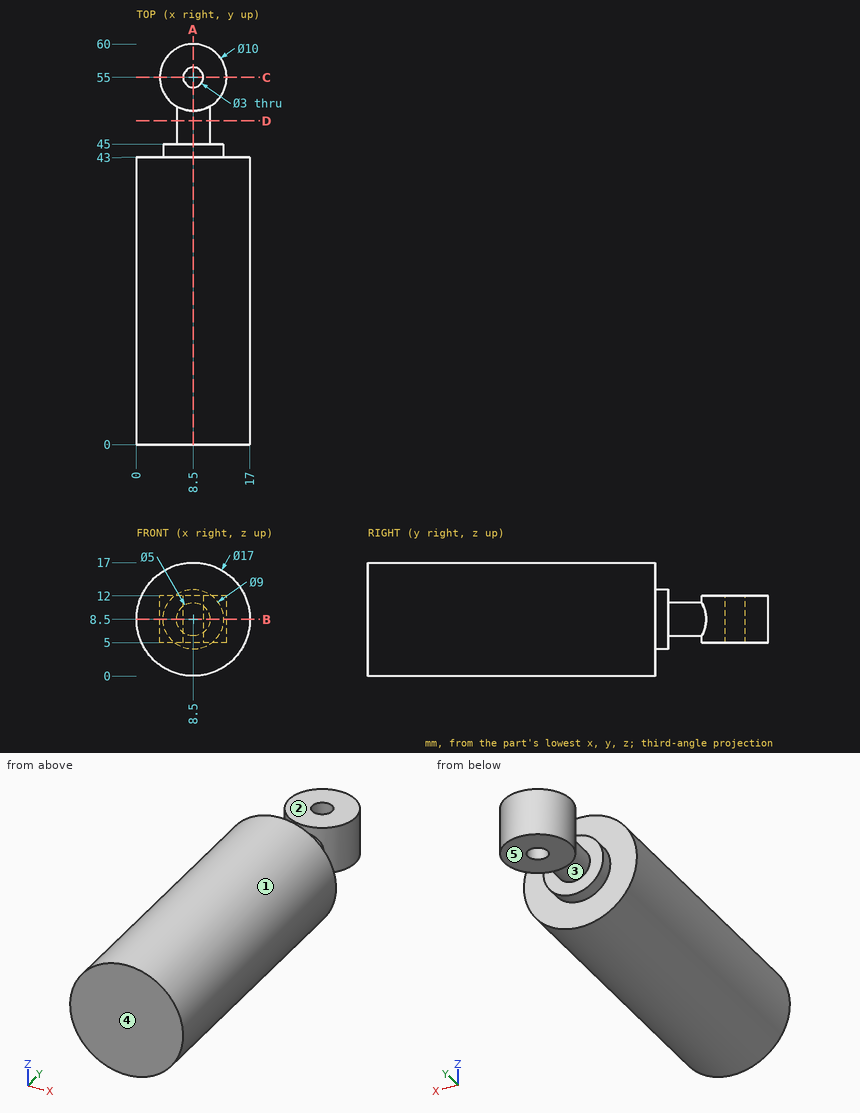
Study the drawing (mm; zero at the part's minimum x, y, z) and answer. A direction names the side the tool comes from. Give positions to 0.01 mm unless a question says otherwise; leave off trailing zeros. Write each loop counter-clockwise with the first axis right and the second up, starting at its lowest first coordinate (ties: lowest second). Pieces come first, ordered by that corner, then holes. Notation, with made-up numbers: (-36.5, 37) - (2.5, 37) arc R12 ccw to (2.5, 45) - close; hole circle Ø2 at (17.25, 69). An arc over 180 degrees is marked (long way). Write item = value, one per line. Start each with the question number.
Item 1: A tool of negligible diameter and unlimited length cuts with its end or side. For the marked faces 1 and 2, from which of +Z, -Z, +X, -X, +Y, -Y can it reach the whole face along a straight path? Write none if from no direction.
Item 2: Find section A-A (x = 8.5). Give the vertices of the cut face in (y, z), then the cut area to 3 significant figures.
Item 3: Each of these flat-tipped pins is pushed along its axis until it touches: P1, Ø3, axis at x = 10, y = 54.5, coming from the -Z side; P2, Ø5, axis at x = 8.5, y = 54, coming from the +Z side; P3, Ø2, axis at y = 27, z = 14.5, coming from the -X side. Where does it stop, or does it pass through?
Item 4: The mould has two halves that part along Y. Classify the marked faces 3, 4 and 5: +Y half, -Y half, draft (parallel to the pull), parting line (faces both ways), or undercut.
Item 5: Find section B-B (z = 8.5). Give the vertices of the cut face in (x, y), then the cut area to 3 significant figures.
Item 6: Find the intervals of material crossed by probe 1 along Y at (x, z) = (8.5, 9.5); probe 2 along Y at (x, z) = (5.5, 11.25); probe 3 along Y at (x, z) = (12, 13.25), in increasing order. Write a range as [from, to].
Item 7: Find section C-C (y = 55). Give the vertices of the cut face in (x, z), then the cut area to 3 significant figures.
Item 8: Find section D-D (y = 48.5). Give the vertices of the cut face in (x, z), then the cut area to 3 significant figures.
Response:
q1.face_1 = +Y, -Y
q1.face_2 = +Z, +X, -X, +Y
q2.outline = (0, 0) - (43, 0) - (43, 4) - (45, 4) - (45, 6) - (50, 6) - (50, 5) - (53.5, 5) - (53.5, 12) - (50, 12) - (50, 11) - (45, 11) - (45, 13) - (43, 13) - (43, 17) - (0, 17) - close; (56.5, 5) - (60, 5) - (60, 12) - (56.5, 12) - close
q2.area = 823 mm²
q3.P1 = 5
q3.P2 = 12
q3.P3 = 1.63
q4.face_3 = undercut
q4.face_4 = -Y half
q4.face_5 = draft
q5.outline = (0, 0) - (17, 0) - (17, 43) - (13, 43) - (13, 45) - (11, 45) - (11, 50.67) arc R5 ccw (long way) to (6, 50.67) - (6, 45) - (4, 45) - (4, 43) - (0, 43) - close; hole circle Ø3 at (8.5, 55)
q5.area = 847 mm²
q6.probe_1 = [0, 53.5], [56.5, 60]
q6.probe_2 = [0, 45], [51, 59]
q6.probe_3 = [0, 43]
q7.outline = (3.5, 5) - (7, 5) - (7, 12) - (3.5, 12) - close; (10, 5) - (13.5, 5) - (13.5, 12) - (10, 12) - close
q7.area = 49.0 mm²
q8.outline = circle Ø5 at (8.5, 8.5)
q8.area = 19.6 mm²
